from build123d import *

# Parameters (mm, degrees)
MAINBASESKETCH_W          = 15.8
MAINBASESKETCH_H          = 3.2
MAINBASEEXTRUDE_DEPTH     = 7.9
MAINBASESHELL_T           = -1.2
UNDERSIDECIRCLEEXT_START  = -0.2
UNDERSIDECIRCLESKETCH_R   = 3.15
UNDERSIDECIRCLESKETCH_R_2 = 2.4
UNDERSIDECIRCLEEXT_DEPTH  = 1.6
CUT_EXTRUDE21_DEPTH       = 19.555463972
SWEEP13_DEPTH             = 3


with BuildPart() as part:
    # MainBaseSketch → MainBaseExtrude (new, symmetric)
    with BuildSketch(Plane.XY):
        with Locations((8.581967213, 1.6)):
            Rectangle(MAINBASESKETCH_W, MAINBASESKETCH_H)
    extrude(amount=MAINBASEEXTRUDE_DEPTH, both=True)

    # MainBaseShell
    mainbaseshell_openings = [part.faces().sort_by_distance(p)[0] for p in [
        (8.581967213, 0, 0),
    ]]
    offset(amount=MAINBASESHELL_T, openings=mainbaseshell_openings, kind=Kind.INTERSECTION)

    # UnderSideCircleSketch → UnderSideCircleExt (add)
    with BuildSketch(Plane.XZ.offset(-2).offset(UNDERSIDECIRCLEEXT_START)):
        with Locations((8.581967213, 0)):
            Circle(UNDERSIDECIRCLESKETCH_R)
        with Locations((8.581967213, 0)):
            Circle(UNDERSIDECIRCLESKETCH_R_2, mode=Mode.SUBTRACT)
    extrude(amount=UNDERSIDECIRCLEEXT_DEPTH)

    # Sketch70 → Cut-Extrude21 (cut, through all)
    with BuildSketch(Plane(origin=(0, 3.2, 0), x_dir=(1, 0, 0), z_dir=(0, 1, 0))):
        with BuildLine():
            Line((8.581967213, 7.9), (16.481967213, 7.9))
            Line((16.481967213, 7.9), (16.481967213, 1.203021508))
            ThreePointArc((16.481967213, 1.203021508), (13.76027584, 6.000468394), (8.581967213, 7.9))
        make_face()
    cut_extrude21 = extrude(amount=-CUT_EXTRUDE21_DEPTH, mode=Mode.SUBTRACT)

    # Mirror7: Cut-Extrude21 across plane
    add(cut_extrude21.mirror(Plane.ZY.offset(-8.581967213)), mode=Mode.SUBTRACT)

    # Sweep8: sweep along a curve in space
    with BuildLine() as sweep8_path:
        Line((15.281967213, 0, -4.27816573), (15.281967213, 2, -4.27816573))
    # Sketch75 → Sweep8 (sweep)
    with BuildSketch(Plane(origin=(0, 0, 0), x_dir=(-1, 0, 0), z_dir=(0, -1, 0))):
        with BuildLine():
            Line((-15.281967213, 4.27816573), (-15.281967213, 0))
            ThreePointArc((-15.281967213, 0), (-15.050769738, 1.744876469), (-14.373133216, 3.369331733))
            Line((-14.373133216, 3.369331733), (-15.281967213, 4.27816573))
        make_face()
        with BuildLine():
            Line((-12.798521236, 6.7), (-11.912237665, 5.813716429))
            ThreePointArc((-11.912237665, 5.813716429), (-10.305060351, 6.474638989), (-8.581967213, 6.7))
            Line((-8.581967213, 6.7), (-12.798521236, 6.7))
        make_face()
    sweep(path=sweep8_path.line)

    # Sweep13: read off the stored shape, not the designer's step
    # Sweep13 outline → Sweep13 (add)
    with BuildSketch(Plane(origin=(0, 0, 0), x_dir=(1, 0, 0), z_dir=(0, 1, 0))):
        with BuildLine():
            ThreePointArc((8.581967213, 6.7), (10.305060351, 6.474638989), (11.912237665, 5.813716429))
            Line((11.912237665, 5.813716429), (12.798521236, 6.7))
            ThreePointArc((12.798521236, 6.7), (8.581967213, 7.9), (4.36541319, 6.7))
            Line((4.36541319, 6.7), (5.249626829, 5.815786361))
            ThreePointArc((5.249626829, 5.815786361), (6.857925652, 6.4759933), (8.581967213, 6.7))
        make_face()
        with BuildLine():
            ThreePointArc((1.881967213, 4.27816573), (1.121797778, 2.803095833), (0.681967213, 1.203021508))
            Line((0.681967213, 1.203021508), (0.681967213, -7.9))
            Line((0.681967213, -7.9), (16.481967213, -7.9))
            Line((16.481967213, -7.9), (16.481967213, 1.203021508))
            ThreePointArc((16.481967213, 1.203021508), (16.042136648, 2.803095833), (15.281967213, 4.27816573))
            Line((15.281967213, 4.27816573), (14.373133216, 3.369331733))
            ThreePointArc((14.373133216, 3.369331733), (15.050769738, 1.744876469), (15.281967213, 0))
            Line((15.281967213, 0), (15.281967213, -6.7))
            Line((15.281967213, -6.7), (1.881967213, -6.7))
            Line((1.881967213, -6.7), (1.881967213, 0))
            ThreePointArc((1.881967213, 0), (2.113164688, 1.744876469), (2.79080121, 3.369331733))
            Line((2.79080121, 3.369331733), (1.881967213, 4.27816573))
        make_face()
    extrude(amount=SWEEP13_DEPTH)


solid = part.part
Part model, mm, in its own coordinate system. A direction names the side the tool comes from. Round coordinates to 2 decimals unless told otherwise and drop trailing zeros. Write each loop counter-clockwise with the first axis right and the second up, starting at its lowest first coordinate (ties: lowest second). Pieces come first, ordered by that corner, then holes. Notation, with made-up numbers: M 22.25,35 L 29.25,35 A29 ccw 29.25,62 Z; hole C 77.25,68.5 d3. An arc over 180 degrees is marked long. Return JSON: item names as keys, results as strings. Group by question number.
(1) Saw through at D-D on z = 2.75. Write the cut outline in (x, y), then the cut area to 3 significant figures.
(2) Which spindle directions (+Z, -Z, +X, -X, +Y, -Y) get a long thin tool onto all of the face, cutting with end or side? Do faces 5 (the face through (9, 0, 7)), 6 (the face through (12.4, 1, -6.3)), 7 (the face through (8, 1, 6.7)), 8 (the face through (8, 2, 7.9)), 9 (the face through (2.34, 0.99, -3.82)). Say none if no direction does.
(3) Pin check, flat tips, straight feed: pin 1 Ø4.5 at (x, z) = (8.58, 0) entering from -Y; pin 2 Ø6.5 at (x, z) = (9.5, -2.5) entering from -Y. Stop position of each tip, or through.
(4) Saw through at C-C on y = 2.95. Write the cut outline in (x, z), then the cut area to 3 significant figures.
(5) Saw through at B-B on x = 9. Write the cut outline in (y, z).
(6) Saw through at A-A on z = 5.5. Write the cut outline in (x, y).
(7) Drill centre lines: probe 1 along X at (y, z) = (1.9, 6.5); probe 2 along X at (y, z) = (1.15, 2.5); probe 3 along Z at (x, y) = (7, 1.05). Where is each one in solid material? Low to high.
(8) Two-plate mould, pull along X, no slides. Class faces 1 (the face through (8, 3.2, 0)), 2 (the face through (4.801, 0.986, -6.264)), 3 (the face through (15.057, 1.014, -1.721)), 4 (the face through (16.482, 2, 3)): +X half, -X half, draft (parallel to the pull), parting line (faces both ways), or undercut.
Returned:
{
 "1": {"outline": "M 0.68,0 L 1.88,0 L 1.88,2 L 7.05,2 L 7.05,0.6 L 10.12,0.6 L 10.12,2 L 15.28,2 L 15.28,0 L 16.48,0 L 16.48,3.2 L 0.68,3.2 Z", "area": "28.1 mm²"},
 "2": {"face 5": "+Z, -Z, +X, -X, -Y", "face 6": "+X, -Y", "face 7": "-Y", "face 8": "+Z, +X, -X, +Y, -Y", "face 9": "-Z, -Y"},
 "3": {"pin 1": "y = 2", "pin 2": "y = 0.6"},
 "4": {"outline": "M 0.68,-1.2 A8.01 ccw 16.48,-1.2 L 16.48,7.9 L 0.68,7.9 Z", "area": "224 mm²"},
 "5": {"outline": "M 0,-7.89 L 3.2,-7.89 L 3.2,7.9 L 0,7.9 L 0,6.7 L 2,6.7 L 2,3.12 L 0.6,3.12 L 0.6,2.36 L 2,2.36 L 2,-2.36 L 0.6,-2.36 L 0.6,-3.12 L 2,-3.12 L 2,-6.69 L 0,-6.69 Z"},
 "6": {"outline": "M 0.68,0 L 1.88,0 L 1.88,2 L 15.28,2 L 15.28,0 L 16.48,0 L 16.48,3.2 L 0.68,3.2 Z"},
 "7": {"probe 1": "0.68 to 1.88, 15.28 to 16.48", "probe 2": "0.68 to 1.88, 6.67 to 10.5, 15.28 to 16.48", "probe 3": "-7.74 to -6.51, -2.72 to -1.8, 1.8 to 2.72, 6.7 to 7.9"},
 "8": {"face 1": "draft", "face 2": "-X half", "face 3": "undercut", "face 4": "+X half"}
}
